The model under review builds one solid part; all positions refer to its coordinate system, in mm. A direction names the side the tool comes from. Coordinates: 2 decimals unless noted, no trailing zeros. Order: outer loops, then holes, each group sorted by start corner. A loop starts at its lowest first (then second) coordinate and runs counter-clockwise, first axis right, second up. Notation, with made-up numbers: M 6,42.5 L 31,42.5 A15 ccw 31,62.5 Z; hole C 12.5,-34 d7. An arc over 180 degrees is marked long. Answer in a Markdown table with one row per item.
from build123d import *

# Parameters (mm, degrees)
SKETCH004_W      = 297
SKETCH004_H      = 75
SKETCH004_R      = 1.6
EXTRUDE004_DEPTH = 1.6
SKETCH005_W      = 28
SKETCH005_H      = 8.6
EXTRUDE005_DEPTH = 10


with BuildPart() as extrude004:
    # Sketch004 → Extrude004 (new body)
    with BuildSketch(Plane.XY.offset(38)):
        with Locations((148.5, 37.5)):
            Rectangle(SKETCH004_W, SKETCH004_H)
        with Locations((6, 69)):
            Circle(SKETCH004_R, mode=Mode.SUBTRACT)
        with Locations((6, 6)):
            Circle(SKETCH004_R, mode=Mode.SUBTRACT)
        with Locations((291, 69)):
            Circle(SKETCH004_R, mode=Mode.SUBTRACT)
        with Locations((291, 6)):
            Circle(SKETCH004_R, mode=Mode.SUBTRACT)
        with Locations((71.45, 69)):
            Circle(SKETCH004_R, mode=Mode.SUBTRACT)
        with Locations((182.245, 6)):
            Circle(SKETCH004_R, mode=Mode.SUBTRACT)
    extrude(amount=EXTRUDE004_DEPTH)


with BuildPart() as obj1:
    # Sketch005 (on Face12 of Extrude004) → Extrude005 (new body)
    with BuildSketch(Plane.XY.offset(39.6)):
        with Locations((187.88, 68.65)):
            Rectangle(SKETCH005_W, SKETCH005_H)
        with Locations((187.88, 57.86)):
            Rectangle(SKETCH005_W, SKETCH005_H)
        with Locations((143.44, 68.65)):
            Rectangle(SKETCH005_W, SKETCH005_H)
        with Locations((143.44, 57.86)):
            Rectangle(SKETCH005_W, SKETCH005_H)
        with Locations((143.44, 41.985)):
            Rectangle(SKETCH005_W, SKETCH005_H)
        with Locations((24.13, 68.65)):
            Rectangle(SKETCH005_W, SKETCH005_H)
        with Locations((273.05, 68.65)):
            Rectangle(SKETCH005_W, SKETCH005_H)
        with Locations((273.05, 41.985)):
            Rectangle(SKETCH005_W, SKETCH005_H)
        with Locations((95.28, 68.65)):
            Rectangle(SKETCH005_W, SKETCH005_H)
        with Locations((95.28, 57.86)):
            Rectangle(SKETCH005_W, SKETCH005_H)
        with Locations((242.252, 68.65)):
            Rectangle(SKETCH005_W, SKETCH005_H)
        with Locations((242.252, 57.86)):
            Rectangle(SKETCH005_W, SKETCH005_H)
        with Locations((242.252, 41.985)):
            Rectangle(SKETCH005_W, SKETCH005_H)
    extrude(amount=EXTRUDE005_DEPTH)

    # Fusion001: union Extrude004
    add(extrude004.part)


solid = obj1.part
(1) Take a section at C-C (y = 19). Write out the cut boundary in (x, z), then the cut area to 3 significant figures.
Report:
| item | result |
|---|---|
| outline | M 0,38 L 297,38 L 297,39.6 L 0,39.6 Z |
| area | 475 mm^2 |
(2) Insertion check: P1, Ø5, axis at x = 239, z = 46.5, coming from the -Y side (3 decimals); P2, Ø3, axis at x = 51.5, y = 64, coming from the +Z side; P3, Ø2, axis at x = 180.5, z = 45, coming from the +Y side; P4, Ø1.5, axis at y = 63, z = 47, coming from the +X side. Each pin has a flat end and moves straight along its axis. Give the tip position at first contact, or say it passes through.
Report:
| item | result |
|---|---|
| P1 | y = 37.685 |
| P2 | z = 39.6 |
| P3 | y = 72.95 |
| P4 | through |
(3) Take a section at B-B (z = 43.5). State how many separate pieces and enclosed holes the cut face has, then the cut area to 3 significant figures.
Report:
| item | result |
|---|---|
| separate pieces | 13 |
| enclosed holes | 0 |
| area | 3,130 mm^2 |
(4) The part is to be moulded in two halves that separate along Y. For faces 4 (the flat face through (242, 53.56, 45)), 5 (the flat face through (242, 72.95, 45)), 6 (the flat face through (273, 64.35, 45)), 7 (the flat face through (259.05, 69, 45)), say which applies: +Y half, -Y half, draft (parallel to the pull), parting line (faces both ways), or undercut.
Report:
| item | result |
|---|---|
| face 4 | undercut |
| face 5 | +Y half |
| face 6 | undercut |
| face 7 | draft |
(5) Take a section at A-A (x = 26.5). Write out the cut boundary in (y, z).
Report:
| item | result |
|---|---|
| outline | M 0,38 L 75,38 L 75,39.6 L 72.95,39.6 L 72.95,49.6 L 64.35,49.6 L 64.35,39.6 L 0,39.6 Z |
(6) Machinability: for faces 1 (the flat face through (242, 37.685, 45)), 2 (the flat face through (242, 64.35, 45)), 3 (the flat face through (157.44, 58, 45)), which of the approach directions +Z, -Z, +X, -X, +Y, -Y give a long, thin tool a straight path to every point of the face, cutting with its end or side? Answer none if there is none.
Report:
| item | result |
|---|---|
| face 1 | +Z, +X, -X, -Y |
| face 2 | +Z, +X, -X |
| face 3 | +Z, +Y, -Y |
(7) Take a section at D-D (x = 233.5). Write out the cut boundary in (y, z) (3 decimals), then the cut area to 3 significant figures.
Report:
| item | result |
|---|---|
| outline | M 0,38 L 75,38 L 75,39.6 L 72.95,39.6 L 72.95,49.6 L 64.35,49.6 L 64.35,39.6 L 62.16,39.6 L 62.16,49.6 L 53.56,49.6 L 53.56,39.6 L 46.285,39.6 L 46.285,49.6 L 37.685,49.6 L 37.685,39.6 L 0,39.6 Z |
| area | 378 mm^2 |
(8) To check wall thickness, follow line 1 (Y direction, x = 291, z = 39); line 2 (X direction, y = 69, z = 39.25); line 3 (X direction, y = 57, z = 44.5). State the ranges of each line that lie inside material, in increasing order. Write a range as [from, to].
Report:
| item | result |
|---|---|
| line 1 | [0, 4.4], [7.6, 67.4], [70.6, 75] |
| line 2 | [0, 4.4], [7.6, 69.85], [73.05, 289.4], [292.6, 297] |
| line 3 | [81.28, 109.28], [129.44, 157.44], [173.88, 201.88], [228.25, 256.25] |
